Work out the finished part from the listing and answer in its coordinate system (mm). Face numbers are marked on the shaded views. Round coordinates to 2 decimals unless told otherwise and drop trailing zeros. Write each loop counter-clockwise with the first axis right and the second up, starting at its lowest first coordinate (ties: lowest second). Pieces come first, ordered by that corner, then holes. Notation, with made-up numbers: (33.5, 83) - (51.5, 83) arc R33 ccw to (51.5, 112) - close; hole circle Ø11 at (-34, 52.5). An arc over 180 degrees is marked (long way). Answer as a JSON object with one key per item and string values.
Autodesk Inventor part; units mm, degrees
ref_plane "YZ Plane" through (0, 0, 0) normal (1, 0, 0) x (0, 1, 0)
ref_plane "XZ Plane" through (0, 0, 0) normal (0, 1, 0) x (-1, 0, 0)
ref_plane "XY Plane" through (0, 0, 0) normal (0, 0, 1) x (1, 0, 0)
sketch "Sketch1" plane through (0, 0, 0) normal (0, 1, 0) x (-1, 0, 0)
  line L0 (0, 0) -> (-30.48, 0)
  line L1 (-30.48, 0) -> (-30.48, -25.4)
  line L2 (-30.48, -25.4) -> (0, -25.4)
  line L3 (0, -25.4) -> (0, 0)
  dimension "d0" = 30.48
  dimension "d1" = 25.4
extrude "Extrusion1" add sketch "Sketch1" along normal blind 15.24
sketch "Sketch4" plane through (30.48, 0, -25.4) normal (0, 0, -1) x (-1, 0, 0)
  circle A0 centre (21.59, 7.62) radius 6.35
  line L0 (30.48, 0) -> (30.48, 15.24)
  dimension "d14" = 12.7
  dimension "d15" = 8.89
extrude "Extrusion4" cut sketch "Sketch4" against normal blind 25.4
sketch "Sketch5" plane through (0, 15.24, 0) normal (0, 1, 0) x (1, 0, 0)
  circle A0 centre (21.59, 12.7) radius 6.35
  line L0 (30.48, 0) -> (30.48, 25.4)
  point P0 (0, 0)
  dimension "d18" = 12.7
  dimension "d19" = 8.89
extrude "Extrusion5" cut sketch "Sketch5" against normal blind 15.24
properties part number "Pivot point"
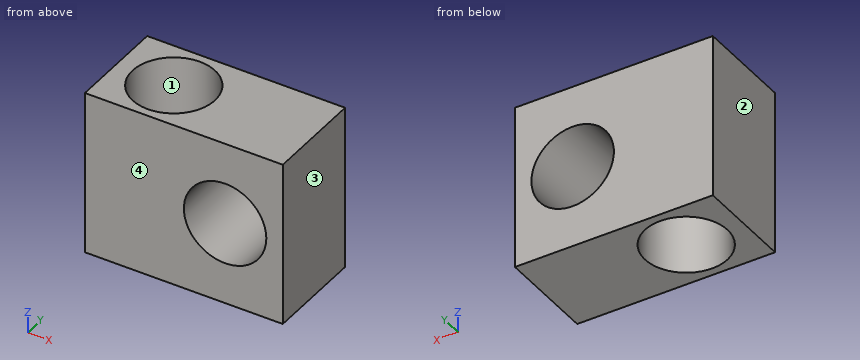
Item 1: Consider line 1 along Y through (x, z) = (8.89, -13.25); line 2 along X through (y, z) = (12, -16.25); line 3 along X through (y, z) = (9, -12.7). Determine where each line is inside the solid, lowest interval first.
Results found:
{"line 1": "0 to 1.27, 13.97 to 15.24", "line 2": "0 to 4.29, 13.49 to 16.33, 26.85 to 30.48", "line 3": "0 to 2.69, 15.09 to 15.24, 27.94 to 30.48"}
Item 2: This flat-tipped pin is pushed along its axis until it touches: P1, Ø10, axis at x = 21.59, z = -12.7, coming from the -Y side. Where does it stop, or does it pass through?
Results found:
{"P1": "through"}
Item 3: A cutting plane is placed at C-C (x = 8.89). Write down the section's boundary in (y, z).
Results found:
{"outline": "(0, -25.4) - (1.27, -25.4) - (1.27, 0) - (0, 0) - close; (13.97, -25.4) - (15.24, -25.4) - (15.24, 0) - (13.97, 0) - close"}
Item 4: Determine the mould class of the marked faces 1, 2, 3 and 4 for opening direction X: pulls with the +X half, pulls with the -X half, needs draft (parallel to the pull), parting line crosses it, or undercut.
Results found:
{"face 1": "undercut", "face 2": "pulls with the -X half", "face 3": "pulls with the +X half", "face 4": "needs draft"}
Item 5: A cutting plane is placed at B-B (y = 7.62). Write down the section's boundary in (x, z).
Results found:
{"outline": "(0, -25.4) - (2.54, -25.4) - (2.54, 0) - (0, 0) - close; (15.24, -25.4) - (30.48, -25.4) - (30.48, 0) - (15.24, 0) - close; hole circle Ø12.7 at (21.59, -12.7)"}
Item 6: A cutting plane is placed at D-D (z = -1.75). Write down the section's boundary in (x, y).
Results found:
{"outline": "(0, 0) - (30.48, 0) - (30.48, 15.24) - (0, 15.24) - close; hole circle Ø12.7 at (8.89, 7.62)"}
Item 7: A cutting plane is placed at A-A (z = -12.7). Write down the section's boundary in (x, y).
Results found:
{"outline": "(0, 0) - (15.24, 0) - (15.24, 15.24) - (0, 15.24) - close; (27.94, 0) - (30.48, 0) - (30.48, 15.24) - (27.94, 15.24) - close; hole circle Ø12.7 at (8.89, 7.62)"}
